Autodesk Inventor part; units mm, degrees
ref_plane "YZ Plane" through (0, 0, 0) normal (1, 0, 0) x (0, 1, 0)
ref_plane "XZ Plane" through (0, 0, 0) normal (0, 1, 0) x (-1, 0, 0)
ref_plane "XY Plane" through (0, 0, 0) normal (0, 0, 1) x (1, 0, 0)
sketch "Sketch1" plane through (0, 0, 0) normal (0, 1, 0) x (-1, 0, 0)
  circle A0 centre (0, 0) radius 9.5
  dimension "d0" = 19
extrude "Extrusion1" add sketch "Sketch1" along normal blind 9
sketch "Sketch2" plane through (0, 0, 0) normal (0, -1, 0) x (1, 0, 0)
  circle A0 centre (0, 0) radius 14
  dimension "d3" = 28
extrude "Extrusion2" add sketch "Sketch2" along normal blind 2
sketch "Sketch5" plane through (0, 0, 0) normal (1, 0, 0) x (0, 1, 0)
  line L0 (-2, 14) -> (-2, -14) construction
  line L1 (-2, 0) -> (-2, 14)
  line L2 (-2, 0) -> (-7, 0)
  circle A0 centre (15.1, 0) radius 22.1 construction
  line L3 (-19.5566, 0) -> (77.1483, 0)
  arc A1 (-2, 14) -> (-7, 0) centre (15.1, 0) ccw
  point P0 (0, 0)
  dimension "d13" = 5
revolve "Revolution1" add sketch "Sketch5" angle 360 about axis through (0, -10, 0) along (0, 1, 0)
sketch "Sketch6" plane through (0, 9, 0) normal (0, 1, 0) x (1, 0, 0)
  point P0 (0, 0)
  point P1 (0, 0)
hole "Hole2" at (0, 9, 0) direction (0, -1, 0) diameter 15 end through all
chamfer "Chamfer2" distance 0.5 angle 45 2 edges at (9.5, 9, 0) (0, 9, -7.5)
properties part number "KN-00-02-06" material "CuZn40"
Model file for the job. Use its own axes, mm. Round coordinates to 2 decimals unless told otherwise and drop trailing zeros. Write each loop counter-clockwise with the first axis right and the second up, starting at its lowest first coordinate (ties: lowest second). Pieces come first, ordered by that corner, then holes. Notation, with made-up numbers: (-27.5, -3.5) - (-11.5, -3.5) arc R4 cw to (-11.5, 0.5) - close; hole circle Ø3 at (-30, 42.25). An arc over 180 degrees is marked (long way). Use CSV: the item, a comma, the result in double quotes. Start each with the question number.
Item 1: Band-saw the part on D-D (z = -10.75). Write the cut outline in (x, y), and give its area (3 significant figures).
Item 2: Band-saw the part on A-A (z = 0). Write the cut outline in (x, y), and give its area (3 significant figures).
Item 3: Band-saw the part on B-B (x = 0). Write the cut outline in (y, z), and give its area (3 significant figures).
Item 4: Two-plate mould, pull along Z, no slides. Class faces 1 (the face through (7.32, 1.31, -1.63)), 2 (the face through (12.932, -0.986, 5.362)), 3 (the face through (-3.3, 0, -9.1)): released by +Z, released by -Z, zero draft, split by the parting line, or undercut.
Item 5: Band-saw the part on C-C (y = 7). Write the cut outline in (x, z).
Item 6: Pin check, flat tips, straight feed: P1, Ø6, axis at x = 2, y = 7.5, coming from the +Z side; P2, Ø4, axis at x = -9, y = 2.5, coming from the -Z side; P3, Ø6, axis at x = 2.5, y = 5, coming from the -Z side. Stop position of each tip, or through.
Item 7: Drill centre lines: L1, parallel to Z at x = 0, y = 3.5; L2, parallel to Z at x = 0, y = -0.5; L3, parallel to X at y = 2.75, z = -2. Where is each one in solid material? Low to high. Write a range as [from, to].
Checked values:
1,outline,"(-8.97, -2) arc R19.31 ccw to (8.97, -2) - (8.97, 0) - (-8.97, 0) - close"
1,area,"62.6 mm²"
2,outline,"(-14, -2) arc R22.1 ccw to (-7.5, -5.69) - (-7.5, 8.5) - (-8, 9) - (-9, 9) - (-9.5, 8.5) - (-9.5, 0) - (-14, 0) - close; (7.5, -5.69) arc R22.1 ccw to (14, -2) - (14, 0) - (9.5, 0) - (9.5, 8.5) - (9, 9) - (8, 9) - (7.5, 8.5) - close"
2,area,"88.7 mm²"
3,outline,"(-5.69, -7.5) arc R22.1 ccw to (-2, -14) - (0, -14) - (0, -9.5) - (8.5, -9.5) - (9, -9) - (9, -8) - (8.5, -7.5) - close; (-5.69, 7.5) - (8.5, 7.5) - (9, 8) - (9, 9) - (8.5, 9.5) - (0, 9.5) - (0, 14) - (-2, 14) arc R22.1 ccw to start"
3,area,"88.7 mm²"
4,face 1,"undercut"
4,face 2,"split by the parting line"
4,face 3,"zero draft"
5,outline,"circle Ø19 at (0, 0); hole circle Ø15 at (0, 0)"
6,P1,"stops at z = 9.5"
6,P2,"stops at z = -6.42"
6,P3,"stops at z = -9.5"
7,L1,"z = [-9.5, -7.5], [7.5, 9.5]"
7,L2,"z = [-14, -7.5], [7.5, 14]"
7,L3,"x = [-9.29, -7.23], [7.23, 9.29]"
